```python
from build123d import *

# Parameters (mm, degrees)
SKETCH1_W               = 2.54
SKETCH1_H               = 2.4
SKETCH1_W_2             = 1.4
SKETCH1_H_2             = 1.45
BOSS_EXTRUDE1_DEPTH     = 4.2
BOSS_EXTRUDE3_START     = -1.2
BOSS_EXTRUDE3_DEPTH     = 0.125
LPATTERN1_START         = -0.125
LPATTERN1_DEPTH         = 0.25
LPATTERN1_2_DEPTH       = 0.25
LPATTERN1_3_DEPTH       = 0.25
LPATTERN1_4_DEPTH       = 0.25
LPATTERN1_START_2       = -4.2
LPATTERN1_5_OUTLINE_W   = 12.7
LPATTERN1_5_OUTLINE_H   = 2.4
LPATTERN1_5_OUTLINE_W_2 = 1.4
LPATTERN1_5_OUTLINE_H_2 = 1.45
LPATTERN1_5_DEPTH       = 8.4
LPATTERN1_6_DEPTH       = 0.25
BOSS_EXTRUDE4_START     = -8.4
SKETCH5_W               = 1.4
SKETCH5_H               = 1.45
SKETCH5_W_2             = 1
SKETCH5_H_2             = 0.4
BOSS_EXTRUDE4_DEPTH     = 8.4
LPATTERN2_COUNT         = 6
LPATTERN2_PITCH         = 2.54


# Read off the part's stored shape, not the designer's step: LPattern1
with BuildPart() as part:
    # Sketch1 → Boss-Extrude1 (new, symmetric)
    with BuildSketch(Plane.XY):
        Rectangle(SKETCH1_W, SKETCH1_H)
        Rectangle(SKETCH1_W_2, SKETCH1_H_2, mode=Mode.SUBTRACT)
    extrude(amount=BOSS_EXTRUDE1_DEPTH, both=True)

    # LPattern1 5 outline → LPattern1 5 (add)
    with BuildSketch(Plane.XY.offset(LPATTERN1_START_2)):
        with Locations((7.62, 0)):
            Rectangle(LPATTERN1_5_OUTLINE_W, LPATTERN1_5_OUTLINE_H)
        with Locations((2.54, 0)):
            Rectangle(LPATTERN1_5_OUTLINE_W_2, LPATTERN1_5_OUTLINE_H_2, mode=Mode.SUBTRACT)
        with Locations((5.08, 0)):
            Rectangle(LPATTERN1_5_OUTLINE_W_2, LPATTERN1_5_OUTLINE_H_2, mode=Mode.SUBTRACT)
        with Locations((7.62, 0)):
            Rectangle(LPATTERN1_5_OUTLINE_W_2, LPATTERN1_5_OUTLINE_H_2, mode=Mode.SUBTRACT)
        with Locations((10.16, 0)):
            Rectangle(LPATTERN1_5_OUTLINE_W_2, LPATTERN1_5_OUTLINE_H_2, mode=Mode.SUBTRACT)
        with Locations((12.7, 0)):
            Rectangle(LPATTERN1_5_OUTLINE_W_2, LPATTERN1_5_OUTLINE_H_2, mode=Mode.SUBTRACT)
    extrude(amount=LPATTERN1_5_DEPTH)



with BuildPart() as body_2:
    # Sketch3 → Boss-Extrude3 (new, symmetric)
    with BuildSketch(Plane(origin=(0, 1.2, 0), x_dir=(1, 0, 0), z_dir=(0, 1, 0)).offset(BOSS_EXTRUDE3_START)):
        with BuildLine():
            Line((-0.914219602, -3.853355377), (-0.914219602, -4.477752268))
            Line((-0.914219602, -4.477752268), (-0.325, -4.477752268))
            Line((-0.325, -4.477752268), (-0.325, -7.045003795))
            ThreePointArc((-0.325, -7.045003795), (0, -7.311534777), (0.325, -7.045003795))
            Line((0.325, -7.045003795), (0.325, -4.477752268))
            Line((0.325, -4.477752268), (0.914219602, -4.477752268))
            Line((0.914219602, -4.477752268), (0.914219602, -3.853355377))
            Line((0.914219602, -3.853355377), (-0.914219602, -3.853355377))
        make_face()
    extrude(amount=BOSS_EXTRUDE3_DEPTH, both=True)


with BuildPart() as body_3:
    # LPattern1 outline → LPattern1 (new body)
    with BuildSketch(Plane(origin=(0, 0, 0), x_dir=(1, 0, 0), z_dir=(0, 1, 0)).offset(LPATTERN1_START)):
        with BuildLine():
            Line((11.074219602, -4.477752268), (11.074219602, -3.853355377))
            Line((11.074219602, -3.853355377), (9.245780398, -3.853355377))
            Line((9.245780398, -3.853355377), (9.245780398, -4.477752268))
            Line((9.245780398, -4.477752268), (9.835, -4.477752268))
            Line((9.835, -4.477752268), (9.835, -7.045003795))
            ThreePointArc((9.835, -7.045003795), (10.16, -7.311534777), (10.485, -7.045003795))
            Line((10.485, -7.045003795), (10.485, -4.477752268))
            Line((10.485, -4.477752268), (11.074219602, -4.477752268))
        make_face()
    extrude(amount=LPATTERN1_DEPTH)


with BuildPart() as body_4:
    # LPattern1 2 outline → LPattern1 2 (new body)
    with BuildSketch(Plane(origin=(0, 0, 0), x_dir=(1, 0, 0), z_dir=(0, 1, 0)).offset(LPATTERN1_START)):
        with BuildLine():
            Line((8.534219602, -4.477752268), (8.534219602, -3.853355377))
            Line((8.534219602, -3.853355377), (6.705780398, -3.853355377))
            Line((6.705780398, -3.853355377), (6.705780398, -4.477752268))
            Line((6.705780398, -4.477752268), (7.295, -4.477752268))
            Line((7.295, -4.477752268), (7.295, -7.045003795))
            ThreePointArc((7.295, -7.045003795), (7.62, -7.311534777), (7.945, -7.045003795))
            Line((7.945, -7.045003795), (7.945, -4.477752268))
            Line((7.945, -4.477752268), (8.534219602, -4.477752268))
        make_face()
    extrude(amount=LPATTERN1_2_DEPTH)


with BuildPart() as body_5:
    # LPattern1 3 outline → LPattern1 3 (new body)
    with BuildSketch(Plane(origin=(0, 0, 0), x_dir=(1, 0, 0), z_dir=(0, 1, 0)).offset(LPATTERN1_START)):
        with BuildLine():
            Line((5.994219602, -4.477752268), (5.994219602, -3.853355377))
            Line((5.994219602, -3.853355377), (4.165780398, -3.853355377))
            Line((4.165780398, -3.853355377), (4.165780398, -4.477752268))
            Line((4.165780398, -4.477752268), (4.755, -4.477752268))
            Line((4.755, -4.477752268), (4.755, -7.045003795))
            ThreePointArc((4.755, -7.045003795), (5.08, -7.311534777), (5.405, -7.045003795))
            Line((5.405, -7.045003795), (5.405, -4.477752268))
            Line((5.405, -4.477752268), (5.994219602, -4.477752268))
        make_face()
    extrude(amount=LPATTERN1_3_DEPTH)


with BuildPart() as body_6:
    # LPattern1 4 outline → LPattern1 4 (new body)
    with BuildSketch(Plane(origin=(0, 0, 0), x_dir=(1, 0, 0), z_dir=(0, 1, 0)).offset(LPATTERN1_START)):
        with BuildLine():
            Line((3.454219602, -4.477752268), (3.454219602, -3.853355377))
            Line((3.454219602, -3.853355377), (1.625780398, -3.853355377))
            Line((1.625780398, -3.853355377), (1.625780398, -4.477752268))
            Line((1.625780398, -4.477752268), (2.215, -4.477752268))
            Line((2.215, -4.477752268), (2.215, -7.045003795))
            ThreePointArc((2.215, -7.045003795), (2.54, -7.311534777), (2.865, -7.045003795))
            Line((2.865, -7.045003795), (2.865, -4.477752268))
            Line((2.865, -4.477752268), (3.454219602, -4.477752268))
        make_face()
    extrude(amount=LPATTERN1_4_DEPTH)


with BuildPart() as body_7:
    # LPattern1 6 outline → LPattern1 6 (new body)
    with BuildSketch(Plane(origin=(0, 0, 0), x_dir=(1, 0, 0), z_dir=(0, 1, 0)).offset(LPATTERN1_START)):
        with BuildLine():
            Line((13.614219602, -4.477752268), (13.614219602, -3.853355377))
            Line((13.614219602, -3.853355377), (11.785780398, -3.853355377))
            Line((11.785780398, -3.853355377), (11.785780398, -4.477752268))
            Line((11.785780398, -4.477752268), (12.375, -4.477752268))
            Line((12.375, -4.477752268), (12.375, -7.045003795))
            ThreePointArc((12.375, -7.045003795), (12.7, -7.311534777), (13.025, -7.045003795))
            Line((13.025, -7.045003795), (13.025, -4.477752268))
            Line((13.025, -4.477752268), (13.614219602, -4.477752268))
        make_face()
    extrude(amount=LPATTERN1_6_DEPTH)


with BuildPart() as part_1:
    add(part.part)

    add(body_7.part)  # Boss-Extrude4 merges body 7
    # Sketch5 → Boss-Extrude4 (add)
    with BuildSketch(Plane(origin=(0, 0, -4.2), x_dir=(-1, 0, 0), z_dir=(0, 0, -1)).offset(BOSS_EXTRUDE4_START)):
        with Locations((-12.7, 0)):
            Rectangle(SKETCH5_W, SKETCH5_H)
        with Locations((-12.7, 0)):
            Rectangle(SKETCH5_W_2, SKETCH5_H_2, mode=Mode.SUBTRACT)
    boss_extrude4 = extrude(amount=BOSS_EXTRUDE4_DEPTH)


    add(body_2.part)  # LPattern2 merges body 2

    add(body_3.part)  # LPattern2 merges body 3

    add(body_4.part)  # LPattern2 merges body 4

    add(body_5.part)  # LPattern2 merges body 5

    add(body_6.part)  # LPattern2 merges body 6
    # LPattern2: Boss-Extrude4 ×6
    with Locations(*[(-i * LPATTERN2_PITCH, 0, 0) for i in range(1, LPATTERN2_COUNT)]):
        add(boss_extrude4)


solid = part_1.part
```
Could you check a few things on this model? Use its own coordinates, in mm. A direction names the side the tool comes from. Round coordinates to 2 decimals unless told otherwise and drop trailing zeros. Write each loop counter-clockwise with the first axis right and the second up, starting at its lowest first coordinate (ties: lowest second). Pieces come first, ordered by that corner, then holes.
(1) Suppose I cut it at D-D on y = 0.5. Write out the boundary of the cut face in (x, z).
Findings below:
outline: (-1.27, -4.2) - (13.97, -4.2) - (13.97, 4.2) - (-1.27, 4.2) - close
(2) If I drill on probe 1 along X at (y, z) = (0, 4.75) (3 decimals); probe 2 along Z at (x, y) = (4.5, -0.2); probe 3 along Y at (x, z) = (7.75, 4.5) (3 decimals), over which ranges is the centre line in solid material (lowest first)?
Findings below:
probe 1: x = -0.325 to 0.325, 2.215 to 2.865, 4.755 to 5.405, 7.295 to 7.945, 9.835 to 10.485, 12.375 to 13.025
probe 2: z = -4.2 to 4.2
probe 3: y = -0.125 to 0.125
(3) Suppose I cut it at C-C on z = 3.5. Write out the boundary of the cut face in (x, y), and give its area (3 significant figures).
Findings below:
outline: (-1.27, -1.2) - (13.97, -1.2) - (13.97, 1.2) - (-1.27, 1.2) - close; hole (-0.5, -0.2) - (0.5, -0.2) - (0.5, 0.2) - (-0.5, 0.2) - close; hole (2.04, -0.2) - (3.04, -0.2) - (3.04, 0.2) - (2.04, 0.2) - close; hole (4.58, -0.2) - (5.58, -0.2) - (5.58, 0.2) - (4.58, 0.2) - close; hole (7.12, -0.2) - (8.12, -0.2) - (8.12, 0.2) - (7.12, 0.2) - close; hole (9.66, -0.2) - (10.66, -0.2) - (10.66, 0.2) - (9.66, 0.2) - close; hole (12.2, -0.2) - (13.2, -0.2) - (13.2, 0.2) - (12.2, 0.2) - close
area: 34.2 mm2
(4) Suppose I cut it at A-A on z = 5. Write out the boundary of the cut face in (x, y) (3 decimals), and give its area (3 significant figures).
Findings below:
outline: (-0.325, -0.125) - (0.325, -0.125) - (0.325, 0.125) - (-0.325, 0.125) - close; (2.215, -0.125) - (2.865, -0.125) - (2.865, 0.125) - (2.215, 0.125) - close; (4.755, -0.125) - (5.405, -0.125) - (5.405, 0.125) - (4.755, 0.125) - close; (7.295, -0.125) - (7.945, -0.125) - (7.945, 0.125) - (7.295, 0.125) - close; (9.835, -0.125) - (10.485, -0.125) - (10.485, 0.125) - (9.835, 0.125) - close; (12.375, -0.125) - (13.025, -0.125) - (13.025, 0.125) - (12.375, 0.125) - close
area: 0.975 mm2
(5) Suppose I cut it at B-B on x = 0.75. Write out the boundary of the cut face in (y, z) (3 decimals).
Findings below:
outline: (-1.2, -4.2) - (1.2, -4.2) - (1.2, 4.2) - (0.125, 4.2) - (0.125, 4.478) - (-0.125, 4.478) - (-0.125, 4.2) - (-1.2, 4.2) - close
(6) Thinking about a two-plate mould opening in Y: for faces 3 (the face through (6, 0, -4.2)), 4 (the face through (5, 0.2, 0)), 5 (the face through (6, 1.2, 0)), which applies, +Y half, -Y half, draft (parallel to the pull), parting line (faces both ways), or undercut?
Findings below:
face 3: draft
face 4: undercut
face 5: +Y half
(7) For pin 1 (1 mm diameter, centred on x = 7, y = 1, fed in from +Z), with a flat end and sliding along its axis, tell me the tip position at first contact or that it passes through.
Findings below:
pin 1: stops at z = 4.2
(8) Which directions (+Z, -Z, +X, -X, +Y, -Y) give clear straight access to the entire face, cutting with the end or side of a thin tool? Please do faces 1 (the face through (13, -0.2, 0)), 2 (the face through (-1.27, 0, 0)).
Findings below:
face 1: +Z, -Z
face 2: +Z, -Z, -X, +Y, -Y
